from build123d import *

# Parameters (mm, degrees)
BOSS_EXTRUDE1_DEPTH = 8
SKETCH1_3_R         = 1.5
BOSS_EXTRUDE2_DEPTH = 6
CUT_EXTRUDE1_START  = 8
SKETCH1_4_R         = 1.5
CUT_EXTRUDE1_DEPTH  = 6


with BuildPart() as part:
    # Sketch1 → Boss-Extrude1 (new body)
    with BuildSketch(Plane.XY):
        Polygon((1.58771324, -2.75), (3.175426481, 0), (1.58771324, 2.75), (-1.58771324, 2.75), (-3.175426481, 0), (-1.58771324, -2.75), align=None)
    extrude(amount=BOSS_EXTRUDE1_DEPTH)

    # Sketch1<3> → Boss-Extrude2 (add)
    with BuildSketch(Plane.XY):
        Circle(SKETCH1_3_R)
    extrude(amount=-BOSS_EXTRUDE2_DEPTH)

    # Sketch1<4> → Cut-Extrude1 (cut)
    with BuildSketch(Plane.XY.offset(CUT_EXTRUDE1_START)):
        Circle(SKETCH1_4_R)
    extrude(amount=-CUT_EXTRUDE1_DEPTH, mode=Mode.SUBTRACT)


solid = part.part
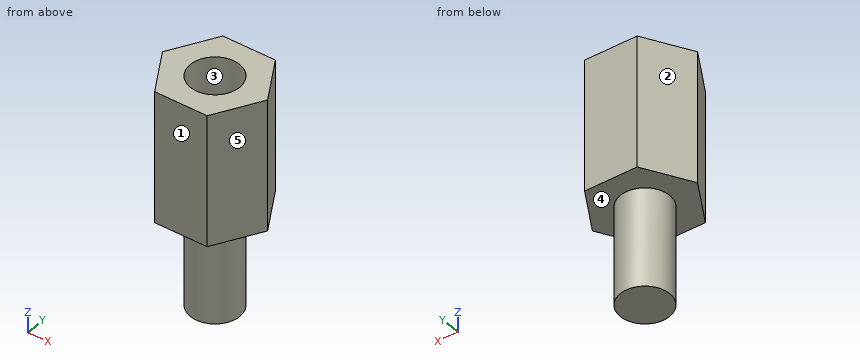
Check sheet for the modelled part. Datum: model origin and axes. Units: mm. Face numbers are marked on the shaded views. A direction names the side the tool comes from. Give positions to 0.01 mm unless a question says otherwise; leave off trailing zeros. Write each loop counter-clockwise with the first axis right and the second up, starting at its lowest first coordinate (ties: lowest second). Pieces come first, ordered by that corner, then holes. Notation, with made-up numbers: (-27.75, -36) -> (-15.75, -36) arc R29 cw to (-15.75, -12) -> close; hole circle Ø5 at (34, -34). An arc over 180 degrees is marked (long way). Write item = value, one per line.
Item 1: Sectioned sample at A-A on z = 3.75. Record the boundary of the cut face in (x, y), and give its area (3 significant figures).
Output:
outline = (-3.18, 0) -> (-1.59, -2.75) -> (1.59, -2.75) -> (3.18, 0) -> (1.59, 2.75) -> (-1.59, 2.75) -> close; hole circle Ø3 at (0, 0)
area = 19.1 mm^2
Item 2: Release check for a two-part mould opening along X. For the marked faces 1, 2 and 3 record: +X half, -X half, draft (parallel to the pull), parting line (faces both ways), or undercut.
Output:
face_1 = draft
face_2 = -X half
face_3 = undercut
Item 3: Sectioned sample at B-B on y = 0.5. Record the boundary of the cut face in (x, z), and give its area (3 significant figures).
Output:
outline = (-2.89, 0) -> (-1.41, 0) -> (-1.41, -6) -> (1.41, -6) -> (1.41, 0) -> (2.89, 0) -> (2.89, 8) -> (1.41, 8) -> (1.41, 2) -> (-1.41, 2) -> (-1.41, 8) -> (-2.89, 8) -> close
area = 46.2 mm^2
Item 4: Gauge pin test, flat ends, axial feed: pin 1 (0.9 mm diameter, centred on x = 0, y = 0, fed in from +Z); pin 2 (1.5 mm diameter, centred on x = 1, z = -2.5, fed in from -Y); pin 3 (2 mm diameter, centred on x = -2, y = 2, fed in from -Z). Record the tip position at first contact, or that the pin passes through.
Output:
pin_1 = 2
pin_2 = -1.48
pin_3 = 0
Item 5: Sectioned sample at C-C on x = 1.25. Record the boundary of the cut face in (y, z).
Output:
outline = (-2.75, 0) -> (-0.83, 0) -> (-0.83, -6) -> (0.83, -6) -> (0.83, 0) -> (2.75, 0) -> (2.75, 8) -> (0.83, 8) -> (0.83, 2) -> (-0.83, 2) -> (-0.83, 8) -> (-2.75, 8) -> close
Item 6: Sectioned sample at D-D on y = -1.7. Record the boundary of the cut face in (x, z), and give its area (3 significant figures).
Output:
outline = (-2.19, 0) -> (2.19, 0) -> (2.19, 8) -> (-2.19, 8) -> close
area = 35.1 mm^2
Item 7: Tool access check on the marked faces 4 and 5. Record the directions out of +Z, -Z, +X, -X, +Y, -Y that give a thin tool (end or side, any length) a straight path to the whole face; none if there is none.
Output:
face_4 = -Z
face_5 = +Z, -Z, +X, -Y
Item 8: Scan lines: probe 1 along Y at (x, z) = (0, 6.3); probe 2 along Z at (x, y) = (-0.25, -1.2); probe 3 along Z at (x, y) = (1, 1.5). Record each from-to range of solid material in increasing order. Write a range as from..to.
Output:
probe_1 = -2.75..-1.5, 1.5..2.75
probe_2 = -6..2
probe_3 = 0..8
